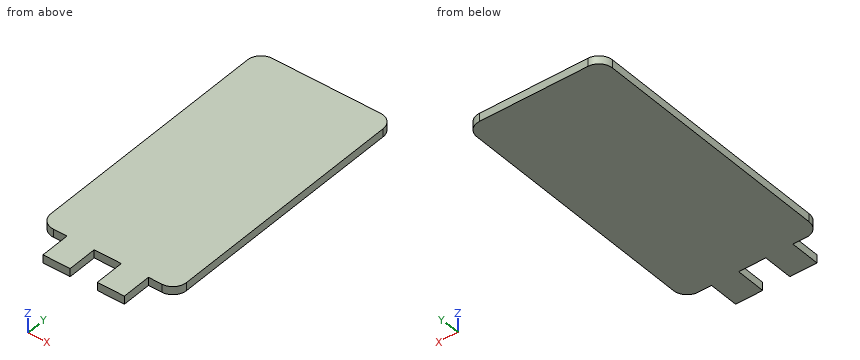
Autodesk Inventor part; units mm, degrees
ref_plane "YZ Plane" through (0, 0, 0) normal (1, 0, 0) x (0, 1, 0)
ref_plane "XZ Plane" through (0, 0, 0) normal (0, 1, 0) x (-1, 0, 0)
ref_plane "XY Plane" through (0, 0, 0) normal (0, 0, 1) x (1, 0, 0)
sketch "Skizze1" plane through (0, 0, 0) normal (0, 0, 1) x (1, 0, 0)
  line L0 (0, 5) -> (0, 95)
  line L1 (5, 100) -> (45, 100)
  line L2 (50, 95) -> (50, 5)
  arc A0 (5, 100) -> (0, 95) centre (5, 95) ccw
  arc A1 (50, 95) -> (45, 100) centre (45, 95) ccw
  arc A2 (45, 0) -> (50, 5) centre (45, 5) ccw
  arc A3 (0, 5) -> (5, 0) centre (5, 5) ccw
  line L3 (10, 0) -> (10, -11)
  line L4 (10, -11) -> (20, -11)
  line L5 (20, -11) -> (20, 0)
  line L6 (30, 0) -> (30, -11)
  line L7 (30, -11) -> (40, -11)
  line L8 (40, -11) -> (40, 0)
  line L9 (5, 0) -> (10, 0)
  line L10 (20, 0) -> (30, 0)
  line L11 (40, 0) -> (45, 0)
  point P0 (0, 0)
  dimension "d1" = 50
  dimension "d3" = 5
  dimension "d4" = 11
  dimension "d5" = 10
  dimension "d6" = 100
extrude "Extrusion1" add sketch "Skizze1" along normal blind 3
properties part number "Scheibe" material "Glas"
Geometry check sheet. Reference: the model listing, model coordinates, mm. Coordinates: 2 decimals unless noted, no trailing zeros. Loops run counter-clockwise (first coordinate to the right, second up) from the corner with the lowest first, then second, coordinate; pieces in that order, holes last. Notation, with made-up numbers: (-18.5, 5.5) - (-14.5, 5.5) arc R19 cw to (-14.5, 21.5) - close; hole circle Ø3 at (-19, -11). An arc over 180 degrees is marked (long way). Use one line per item in the form item = value. Start each with the question number.
Item 1: Gauge pin test, flat ends, axial feed: pin 1 (0.9 mm diameter, centred on x = 8.5, z = 1, fed in from -Y); pin 2 (0.9 mm diameter, centred on y = -8, z = 1, fed in from -X); pin 3 (0.9 mm diameter, centred on y = -3.5, z = 1, fed in from +X). Record the tip position at first contact, or that the pin passes through.
Item 2: Section check A-A, the plane z = 1.75. Enter the section's corners in (x, y).
Item 3: Thickness scan on probe 1 along X at (y, z) = (-1.5, 2.1); probe 2 along Y at (x, z) = (44, 1.3); probe 3 along Y at (x, z) = (4, 2.8). Record the ranges inside material, lowest first.
Computed:
q1.pin_1 = 0
q1.pin_2 = 10
q1.pin_3 = 40
q2.outline = (0, 5) arc R5 ccw to (5, 0) - (10, 0) - (10, -11) - (20, -11) - (20, 0) - (30, 0) - (30, -11) - (40, -11) - (40, 0) - (45, 0) arc R5 ccw to (50, 5) - (50, 95) arc R5 ccw to (45, 100) - (5, 100) arc R5 ccw to (0, 95) - close
q3.probe_1 = 10 to 20, 30 to 40
q3.probe_2 = 0 to 100
q3.probe_3 = 0.1 to 99.9
